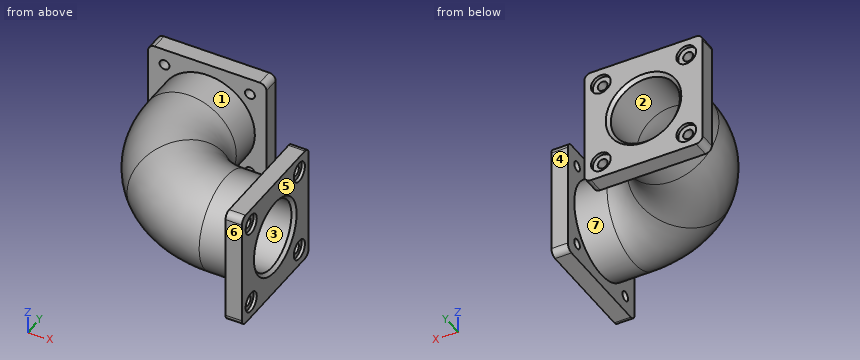
from build123d import *
from build123d.topology import SkipClean

# Parameters (mm, degrees)
BOSS_EXTRUDE1_DEPTH = 50
SKETCH2_R           = 30
CUT_EXTRUDE1_DEPTH  = 10
SKETCH5_R           = 15
CUT_EXTRUDE2_DEPTH  = 258.681974535
SKETCH6_R           = 145
BOSS_EXTRUDE3_DEPTH = 100
SKETCH7_R           = 105
CUT_EXTRUDE3_DEPTH  = 296.465734054
CHAMFER1_SIZE       = 10
SWEEP1_OUTLINE_R    = 145
SWEEP1_OUTLINE_R_2  = 105
SWEEP1_ANGLE        = 45


# Read off the part's stored shape, not the designer's step: Sweep1
with BuildPart() as part:
    # Sketch1 → Boss-Extrude1 (new body)
    with BuildSketch(Plane(origin=(0, 0, 0), x_dir=(0, 0, -1), z_dir=(1, 0, 0))):
        with BuildLine():
            Line((-160, 180), (160, 180))
            ThreePointArc((160, 180), (174.142135624, 174.142135624), (180, 160))
            Line((180, 160), (180, -160))
            ThreePointArc((180, -160), (174.142135624, -174.142135624), (160, -180))
            Line((160, -180), (-160, -180))
            ThreePointArc((-160, -180), (-174.142135624, -174.142135624), (-180, -160))
            Line((-180, -160), (-180, 160))
            ThreePointArc((-180, 160), (-174.142135624, 174.142135624), (-160, 180))
        make_face()
    extrude(amount=-BOSS_EXTRUDE1_DEPTH)

    # Sketch2 → Cut-Extrude1 (cut)
    with BuildSketch(Plane(origin=(0, 0, 0), x_dir=(0, 0, -1), z_dir=(1, 0, 0))):
        with Locations((-130, 130)):
            Circle(SKETCH2_R)
        with Locations((130, 130)):
            Circle(SKETCH2_R)
        with Locations((130, -130)):
            Circle(SKETCH2_R)
        with Locations((-130, -130)):
            Circle(SKETCH2_R)
    extrude(amount=-CUT_EXTRUDE1_DEPTH, mode=Mode.SUBTRACT)

    # Sketch5 → Cut-Extrude2 (cut, through all)
    with BuildSketch(Plane(origin=(-10, 0, 0), x_dir=(0, 0, -1), z_dir=(1, 0, 0))):
        with Locations((-130, 130)):
            Circle(SKETCH5_R)
        with Locations((130, 130)):
            Circle(SKETCH5_R)
        with Locations((130, -130)):
            Circle(SKETCH5_R)
        with Locations((-130, -130)):
            Circle(SKETCH5_R)
    extrude(amount=-CUT_EXTRUDE2_DEPTH, mode=Mode.SUBTRACT)

    # Sketch6 → Boss-Extrude3 (add)
    with BuildSketch(Plane.ZY.offset(50)):
        with Locations(Location((0, 0, 0), (0, 0, 180))):
            Circle(SKETCH6_R)
    extrude(amount=BOSS_EXTRUDE3_DEPTH)

    # Sketch7 → Cut-Extrude3 (cut, through all)
    with BuildSketch(Plane(origin=(0, 0, 0), x_dir=(0, 0, -1), z_dir=(1, 0, 0))):
        Circle(SKETCH7_R)
    extrude(amount=-CUT_EXTRUDE3_DEPTH, mode=Mode.SUBTRACT)

    # Chamfer1
    chamfer1_edges = [part.edges().sort_by_distance(p)[0] for p in [
        (0, 0, 105),
    ]]
    chamfer(chamfer1_edges, length=CHAMFER1_SIZE)

    # Sweep1 outline → Sweep1 (revolve)
    with BuildSketch(Plane(origin=(-150, 260, 0), x_dir=(-0.707106781186543, -0.707106781186552, 0), z_dir=(-0.707106781186552, 0.707106781186543, 0))):
        with Locations((260, 0)):
            Circle(SWEEP1_OUTLINE_R)
        with Locations((260, 0)):
            Circle(SWEEP1_OUTLINE_R_2, mode=Mode.SUBTRACT)
    revolve(axis=Axis((-150, 260, 0), (0, 0, 1)), revolution_arc=SWEEP1_ANGLE)

    # Mirror3: part across plane


with BuildPart() as part_1:
    with SkipClean():  # the faces are left unmerged after this step: merging them gives an invalid solid
        add(part.part)
        add(part.part.mirror(Plane(origin=(-333.847763109, 76.152236891, 0), x_dir=(0, 0, 1), z_dir=(-0.7071067811865515, 0.7071067811865437, 0))))


solid = part_1.part
The listing builds one solid part. Answer for the finished solid, in the listing's coordinates (mm). Face numbers are marked on the shaded views. A direction names the side the tool comes from. Give positions to 0.01 mm unless a question says otherwise; leave off trailing zeros. Order: outer loops, then holes, each group sorted by start corner. A loop starts at its lowest first (then second) coordinate and runs counter-clockwise, first axis right, second up. Notation, with made-up numbers: (24.5, -34) - (40.5, -34) arc R33 cw to (40.5, 3) - close; hole circle Ø9 at (47.25, -32.5). An arc over 180 degrees is marked (long way). One line per item, written item: value. Start each with the question number.
1) A tool of negligible diameter and unlimited length cuts with its end or side. For the marked faces 1, 2, 3 and 4, from which of +Z, -Z, +X, -X, +Y, -Y can it reach the whole face along a straight path? Write none if from no direction.
2) Find the intervals of material crossed by L1, parallel to X at y = 407, z = -130; L2, parallel to Y at x = -236, z = 36.5; L3, parallel to Y at x = -256, z = 70, in increasing order.
3) A cutting plane is placed at A-A on y = 312. Give the vertices of the cut face in (x, z).
4) The mould has two halves that part along X. Classify the marked faces 5, 6 and 7: released by +X, released by -X, zero draft, split by the parting line, or undercut.
5) Given pin 1 Ø15 at (y, z) = (397.5, 30.5) entering from +X; pin 2 Ø18 at (x, z) = (-549, 125.5) entering from +Y; pin 3 Ø4 at (x, z) = (-205, -55.5) entering from -Y, each flat-ended and moving along its own axis, determine where each tip first touches the part or whether it passes through.
6) A cutting plane is placed at B-B on z = 130. State how many separate pieces and enclosed holes the cut face has, then the cut area to 3 significant figures.
Answer sheet:
1. face 1: none
1. face 2: +Y
1. face 3: +X
1. face 4: +Z, -Z, +X, +Y
2. L1: x = -590 to -570, -510 to -310, -250 to -230
2. L2: y = -130.98 to -87.98, 123.25 to 176.79, 360 to 410
2. L3: y = -112.18 to -61.22, 112.38 to 179.64, 360 to 410
3. outline: circle Ø290 at (-410, 0); hole circle Ø210 at (-410, 0)
4. face 5: released by +X
4. face 6: zero draft
4. face 7: undercut
5. pin 1: stops at x = -230
5. pin 2: stops at y = 400
5. pin 3: stops at y = -130.97
6. separate pieces: 5
6. enclosed holes: 0
6. area: 107,000 mm2
